Here's the drawing with two shaded views (mm, measured from the low corner). I have some questions. A direction names the side the tool comes from. Coordinates: 2 decimals unless noted, no trailing zeros. Write each loop counter-clockwise with the first axis right and the second up, starting at its lowest first coordinate (ties: lowest second). Pieces come first, ordered by that corner, then holes. Notation, with made-up numbers: (49, -22) -> (89, -22) arc R16 cw to (89, 0) -> close; hole circle Ø11 at (-16.5, -23.75). An arc over 180 degrees is marked (long way). Put each result on its own line as item: value. Start each with the question number.
Item 1: If we mould it in two halves opening along Z, with no side actions, what happens to the marked faces 3, 4, 5 and 6? For each: released by +Z, released by -Z, zero draft, split by the parting line, or undercut.
Item 2: I want a section at D-D, the plane z = 7.5. List the corners of the cut face in (x, y) for me.
Item 3: For pin 1 (1 mm diameter, centred on x = 14.5, y = 4.5, fed in from -Z); pin 2 (2 mm diameter, centred on x = 3, z = 7.1, fed in from +Y); pin 3 (2 mm diameter, centred on y = 1.5, z = 2.5, fed in from +X), each with a flat end and sliding along its axis, tell me the tip position at first contact or that it passes through.
Item 4: On a 3-axis mill with a long thin cutter (end or side, diameter ignored), from which of +Z, -Z, +X, -X, +Y, -Y can I reach the whole of each face in a straight line? I mean the marked faces 1 and 2. Say none if no direction works.
Item 5: I need wall thicknesses on line 1 (Z direction, x = 17.5, y = 1.45); line 2 (X direction, y = 1.4, z = 3); line 3 (X direction, y = 0.8, z = 11). Which ranges of each line are inside material? Lowest first, please. Write a range as [from, to].
Item 6: I want a section at C-C, the plane y = 1.3. State how many separate pieces and enclosed holes the cut face has, then the cut area to 3 significant figures.
Item 7: I want a section at A-A, the plane x = 10.5. List the corners of the cut face in (y, z) for me, then the cut area to 3 significant figures.
Item 8: I want a section at B-B, the plane z = 10.5. List the corners of the cut face in (x, y) for me.
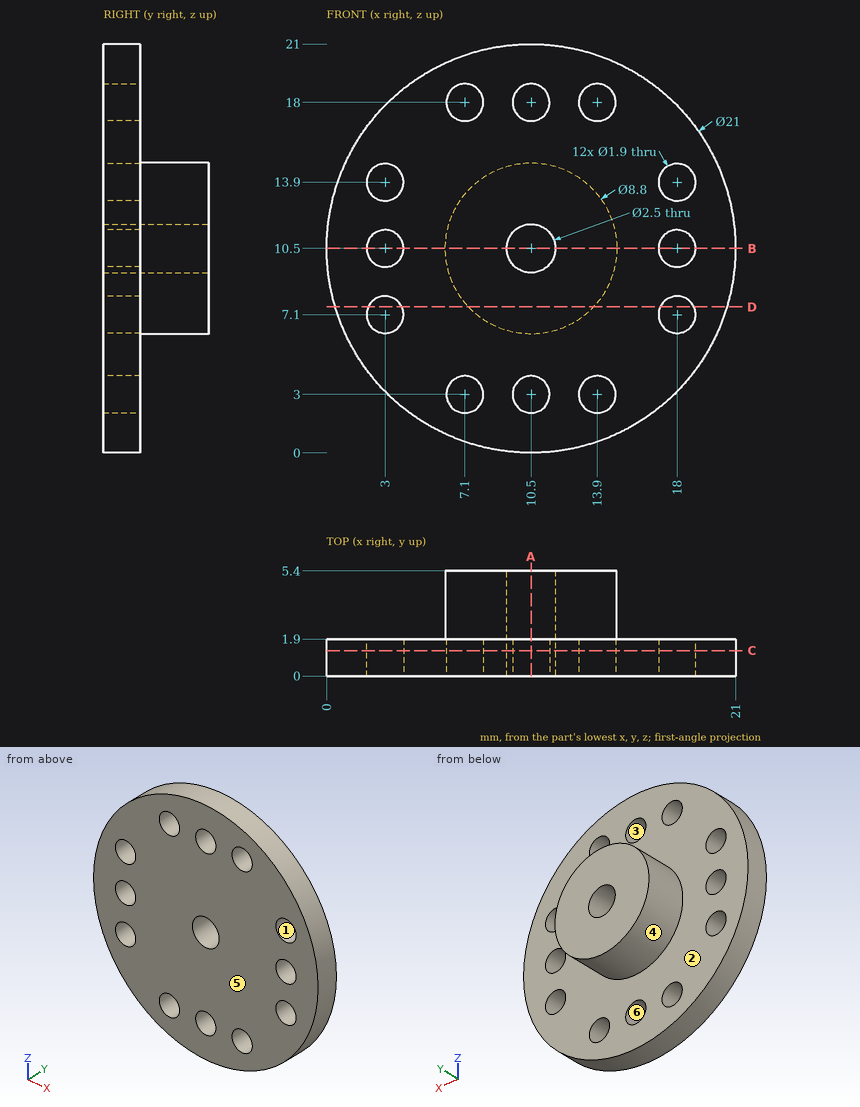
Calculated:
1. face 3: undercut
1. face 4: split by the parting line
1. face 5: zero draft
1. face 6: undercut
2. outline: (0.44, 0) -> (2.14, 0) -> (2.14, 1.9) -> (0.44, 1.9) -> close; (3.86, 0) -> (17.14, 0) -> (17.14, 1.9) -> (13.72, 1.9) -> (13.72, 5.4) -> (7.28, 5.4) -> (7.28, 1.9) -> (3.86, 1.9) -> close; (18.86, 0) -> (20.56, 0) -> (20.56, 1.9) -> (18.86, 1.9) -> close
3. pin 1: stops at z = 7.83
3. pin 2: stops at y = 1.9
3. pin 3: stops at x = 18.33
4. face 1: +Y, -Y
4. face 2: +Y
5. line 1: z = [2.67, 6.29], [7.91, 9.69], [11.31, 13.09], [14.71, 18.33]
5. line 2: x = [3.15, 6.15], [8.05, 9.55], [11.45, 12.95], [14.85, 17.85]
5. line 3: x = [0.01, 2.19], [3.81, 9.35], [11.65, 17.19], [18.81, 20.99]
6. separate pieces: 1
6. enclosed holes: 13
6. area: 307 mm2
7. outline: (0, 0) -> (1.9, 0) -> (1.9, 2.05) -> (0, 2.05) -> close; (0, 3.95) -> (1.9, 3.95) -> (1.9, 6.1) -> (5.4, 6.1) -> (5.4, 9.25) -> (0, 9.25) -> close; (0, 11.75) -> (5.4, 11.75) -> (5.4, 14.9) -> (1.9, 14.9) -> (1.9, 17.05) -> (0, 17.05) -> close; (0, 18.95) -> (1.9, 18.95) -> (1.9, 21) -> (0, 21) -> close
7. area: 50.0 mm2
8. outline: (0, 0) -> (2.05, 0) -> (2.05, 1.9) -> (0, 1.9) -> close; (3.95, 0) -> (9.25, 0) -> (9.25, 5.4) -> (6.1, 5.4) -> (6.1, 1.9) -> (3.95, 1.9) -> close; (11.75, 0) -> (17.05, 0) -> (17.05, 1.9) -> (14.9, 1.9) -> (14.9, 5.4) -> (11.75, 5.4) -> close; (18.95, 0) -> (21, 0) -> (21, 1.9) -> (18.95, 1.9) -> close
